The drawing under review shows one solid part. Ordinate dimensions are in mm from its lowest x, y, z. A direction names the side the tool comes from. Give positions to 0.01 mm unless a question says otherwise; leave off trailing zeros. Write each loop counter-clockwise with the first axis right and the second up, starting at its lowest first coordinate (ties: lowest second). Pieces come first, ordered by that corner, then holes. Notation, with made-up numbers: (71.5, 16) -> (112.5, 16) arc R18 ccw to (112.5, 37) -> close; hole circle Ø9 at (-6.5, 1.25). An arc over 180 degrees is marked (long way). Write item = value, one per line.
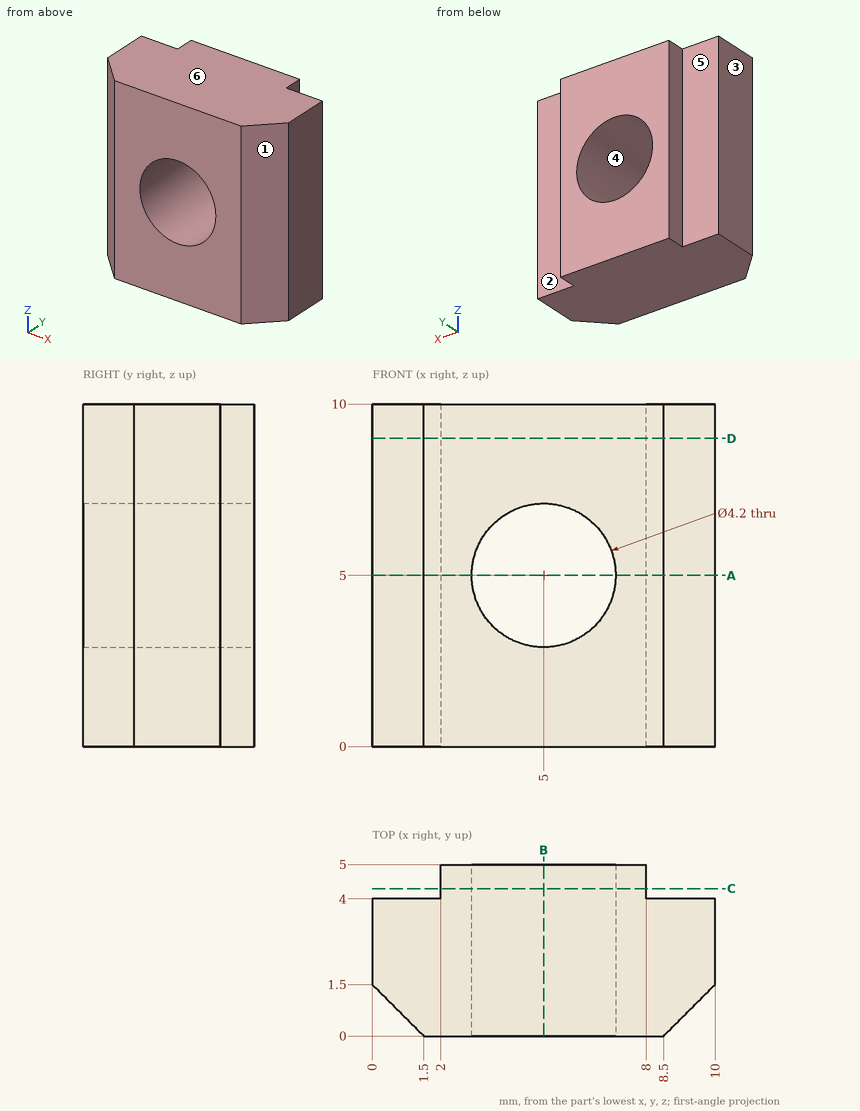
(1) Take a section at A-A (z = 5). Write out the cut boundary in (x, y).
Answers below:
outline = (0, 1.5) -> (1.5, 0) -> (2.9, 0) -> (2.9, 5) -> (2, 5) -> (2, 4) -> (0, 4) -> close; (7.1, 0) -> (8.5, 0) -> (10, 1.5) -> (10, 4) -> (8, 4) -> (8, 5) -> (7.1, 5) -> close
(2) For pin 1 (0.8 mm diameter, centred on y = 4.5, z = 4, fed in from -X); pin 2 (1.6 mm diameter, centred on x = 1, z = 5, fed in from +Y), all flat-tipped, find the tip position at first contact; note any pin that passes through.
Answers below:
pin_1 = 2
pin_2 = 4
(3) The part is to be moulded in two halves that separate along X. For the marked faces 1, 2, 3 and 4, say which applies: released by +X, released by -X, zero draft, split by the parting line, or undercut.
Answers below:
face_1 = released by +X
face_2 = zero draft
face_3 = released by -X
face_4 = undercut
(4) To check wall thickness, follow probe 1 along X at (y, z) = (2.9, 5); probe 2 along X at (y, z) = (2.2, 6.5). State the ranges of each line that lie inside material, in increasing order.
Answers below:
probe_1 = 0 to 2.9, 7.1 to 10
probe_2 = 0 to 3.53, 6.47 to 10
(5) Tool access review of the marked faces 5 and 6: name each direction out of +Z, -Z, +X, -X, +Y, -Y from which nothing blocks a thin tool from reaching the whole face with its end or side.
Answers below:
face_5 = +Z, -Z, -X, +Y
face_6 = +Z, +X, -X, +Y, -Y
(6) Take a section at D-D (z = 9). Write out the cut boundary in (x, y), plus the area to 4 significant figures.
Answers below:
outline = (0, 1.5) -> (1.5, 0) -> (8.5, 0) -> (10, 1.5) -> (10, 4) -> (8, 4) -> (8, 5) -> (2, 5) -> (2, 4) -> (0, 4) -> close
area = 43.75 mm^2
(7) Take a section at C-C (y = 4.3). Write out the cut boundary in (x, z).
Answers below:
outline = (2, 0) -> (8, 0) -> (8, 10) -> (2, 10) -> close; hole circle Ø4.2 at (5, 5)
(8) Take a section at B-B (x = 5). Write out the cut boundary in (y, z), plus the area to 3 significant figures.
Answers below:
outline = (0, 0) -> (5, 0) -> (5, 2.9) -> (0, 2.9) -> close; (0, 7.1) -> (5, 7.1) -> (5, 10) -> (0, 10) -> close
area = 29.0 mm^2
